Work out the finished part from the listing and answer in its coordinate system (mm). A direction names the side the tool comes from. Coordinates: 2 decimals unless noted, no trailing zeros. Write each loop counter-clockwise with the first axis right and the second up, starting at its lowest first coordinate (ties: lowest second). Pieces come first, ordered by that corner, then holes. Notation, with made-up numbers: (38, -39) - (77, -39) arc R16 cw to (77, -35) - close; hole circle Ø10 at (13, 73). An arc over 180 degrees is marked (long way). One line per item, written item: value.
Autodesk Inventor part; units mm, degrees
ref_plane "YZ Plane" through (0, 0, 0) normal (1, 0, 0) x (0, 1, 0)
ref_plane "XZ Plane" through (0, 0, 0) normal (0, 1, 0) x (-1, 0, 0)
ref_plane "XY Plane" through (0, 0, 0) normal (0, 0, 1) x (1, 0, 0)
sketch "Sketch1" plane through (0, 0, 0) normal (0, 0, 1) x (1, 0, 0)
  line L0 (0, 0) -> (25.4, 0)
  line L1 (25.4, 0) -> (25.4, 50.8)
  line L2 (25.4, 50.8) -> (0, 50.8)
  line L3 (0, 50.8) -> (0, 0)
  line L4 (3.175, 3.175) -> (22.225, 3.175)
  line L5 (22.225, 3.175) -> (22.225, 47.625)
  line L6 (22.225, 47.625) -> (3.175, 47.625)
  line L7 (3.175, 47.625) -> (3.175, 3.175)
  dimension "d0" = 50.8
  dimension "d1" = 25.4
  dimension "d2" = 3.175
  dimension "d3" = 3.175
  dimension "d4" = 3.175
  dimension "d5" = 3.175
extrude "Extrusion1" add sketch "Sketch1" along normal blind 685.8
sketch "Sketch2" plane through (0, 50.8, 0) normal (0, 1, 0) x (1, 0, 0)
  line L0 (25.4, 0) -> (25.4, -685.8)
  line L1 (25.4, 0) -> (0, 0)
  circle A0 centre (12.7, -12.7) radius 3.175
  dimension "d8" = 6.35
  dimension "d9" = 12.7
  dimension "d10" = 12.7
extrude "Extrusion2" cut sketch "Sketch2" against normal through all
pattern_linear "Rectangular Pattern1" count 27 spacing 25.4 along (0, 0, 1) of "Extrusion2"
properties part number "OuterCrossRail" material "Aluminum-6061"
Item 1: Consider probe 1 along X at (y, z) = (1.75, 469.9) (3 decimals); probe 2 along Y at (x, z) = (8.25, 316) (3 decimals); probe 3 along X at (y, z) = (11, 538) (3 decimals). Determine where each line is inside the solid, lowest interval first.
Evaluation:
probe 1: x = 0 to 9.525, 15.875 to 25.4
probe 2: y = 0 to 3.175, 47.625 to 50.8
probe 3: x = 0 to 3.175, 22.225 to 25.4
Item 2: Given pin 1 (4 mm diameter, centred on x = 12.7, z = 393.7, fed in from -Y), flat-ended and moving along its own axis, determine where the tip first touches the part or whether it passes through.
Evaluation:
pin 1: passes through
Item 3: Which of the six approach directions +Z, -Z, +X, -X, +Y, -Y give full straight-line access (tool end or side, diameter ignored) to faces 1 (the face through (13, 3.175, 338)), 2 (the face through (2, 24, 0))?
Evaluation:
face 1: +Z, -Z
face 2: -Z, +X, -X, +Y, -Y
Item 4: Section A-A, the plane y = 26.5 is taken. Determine the outline of the cut face in (x, z) (3 decimals).
Evaluation:
outline: (0, 0) - (3.175, 0) - (3.175, 685.8) - (0, 685.8) - close; (22.225, 0) - (25.4, 0) - (25.4, 685.8) - (22.225, 685.8) - close
Item 5: Determine the mould class of faces 3 (the face through (2, 24, 685.8)), 4 (the face through (13, 0, 338)), 5 (the face through (13, 47.625, 338)) for opening direction Y: +Y half, -Y half, draft (parallel to the pull), parting line (faces both ways), or undercut.
Evaluation:
face 3: draft
face 4: -Y half
face 5: undercut
Item 6: Section B-B, the plane z = 434.5 is taken. Determine the outline of the cut face in (x, y) (3 decimals), then the cut area to 3 significant figures.
Evaluation:
outline: (0, 0) - (25.4, 0) - (25.4, 50.8) - (0, 50.8) - close; hole (3.175, 3.175) - (22.225, 3.175) - (22.225, 47.625) - (3.175, 47.625) - close
area: 444 mm2
